```python
from build123d import *

# Parameters (mm, degrees)
SKETCH_R      = 6
SKETCH_R_2    = 2.1
PAD_DEPTH     = 7
SKETCH001_R   = 9
SKETCH001_R_2 = 2.1
PAD001_DEPTH  = 1
SKETCH002_R   = 9
SKETCH002_R_2 = 2.1
PAD002_DEPTH  = 1


with BuildPart() as part:
    # Sketch → Pad (new body)
    with BuildSketch(Plane.XY):
        Circle(SKETCH_R)
        Circle(SKETCH_R_2, mode=Mode.SUBTRACT)
    extrude(amount=PAD_DEPTH)

    # Sketch001 (on Face4 of Pad) → Pad001 (join)
    with BuildSketch(Plane.XY.offset(7)):
        Circle(SKETCH001_R)
        Circle(SKETCH001_R_2, mode=Mode.SUBTRACT)
    extrude(amount=PAD001_DEPTH)

    # Sketch002 (on Face2 of Pad001) → Pad002 (join)
    with BuildSketch(Plane(origin=(0, 0, 0), x_dir=(1, 0, 0), z_dir=(0, 0, -1))):
        Circle(SKETCH002_R)
        Circle(SKETCH002_R_2, mode=Mode.SUBTRACT)
    extrude(amount=PAD002_DEPTH)


solid = part.part
```
Source: CAD feature listing. Evaluate the final solid. Frame: model axes, mm. A direction names the side the tool comes from. Round coordinates to 2 decimals unless told otherwise and drop trailing zeros. Order: outer loops, then holes, each group sorted by start corner. A loop starts at its lowest first (then second) coordinate and runs counter-clockwise, first axis right, second up. Notation, with made-up numbers: (87, 22) -> (146, 22) arc R27 cw to (146, 52) -> close; hole circle Ø4 at (-11, 3.5). An arc over 180 degrees is marked (long way). One line per item, written item: value. Start each with the question number.
Q1. Section query A-A (x = 0). Return the cut outline in (y, z).
Q2. Material intervals for probe 1 along Z at (x, y) = (-1, 8); probe 2 along Y at (x, z) = (0, 5.25); probe 3 along Y at (x, z) = (-0.5, 2), sorted ascending.
Q3. Section query C-C (z = 5). Return the cut outline in (x, y), plus the area to 3 significant figures.
Q4. Pin query (flat end, axial travel): pin 1 (2 mm diameter, centred on y = 5.5, z = 3.5, fed in from +X); pin 2 (3 mm diameter, centred on y = 4.5, z = 6, fed in from -X); pin 3 (1.5 mm diameter, centred on x = -2.5, z = 0, fed in from -Y). Return the tip coordinate at first contact, or that it passes through.
Q5. Draft query along Z for faces 1 (the cylindrical face through (-6, 0, 3)), 2 (the cylindrical face through (-1.172, 8.923, 7.493)), 3 (the flat face through (2, 2, -1)). Return one class per face: pulls with the +Z half, pulls with the -Z half, needs draft (parallel to the pull), parting line crosses it, or undercut.
Q6. Section query D-D (x = 4.25). Return the cut outline in (y, z), plus the area to 3 significant figures.
Q7. Access query for faces 4 (the flat face through (2, -2, 8)), 5 (the flat face through (2, 6, 0)). Directions: +Z, -Z, +X, -X, +Y, -Y. A direction counts if a zero-diameter tool reaches every point of the face in a straight line with its end or side. Return the directions, or none.
Findings below:
1. outline: (-9, -1) -> (-2.1, -1) -> (-2.1, 8) -> (-9, 8) -> (-9, 7) -> (-6, 7) -> (-6, 0) -> (-9, 0) -> close; (2.1, -1) -> (9, -1) -> (9, 0) -> (6, 0) -> (6, 7) -> (9, 7) -> (9, 8) -> (2.1, 8) -> close
2. probe 1: -1 to 0, 7 to 8
2. probe 2: -6 to -2.1, 2.1 to 6
2. probe 3: -5.98 to -2.04, 2.04 to 5.98
3. outline: circle Ø12 at (0, 0); hole circle Ø4.2 at (0, 0)
3. area: 99.2 mm²
4. pin 1: x = 3.97
4. pin 2: x = -8.34
4. pin 3: y = -8.83
5. face 1: undercut
5. face 2: needs draft
5. face 3: pulls with the -Z half
6. outline: (-7.93, -1) -> (7.93, -1) -> (7.93, 0) -> (4.24, 0) -> (4.24, 7) -> (7.93, 7) -> (7.93, 8) -> (-7.93, 8) -> (-7.93, 7) -> (-4.24, 7) -> (-4.24, 0) -> (-7.93, 0) -> close
6. area: 91.0 mm²
7. face 4: +Z, +X, -X, +Y, -Y
7. face 5: none
